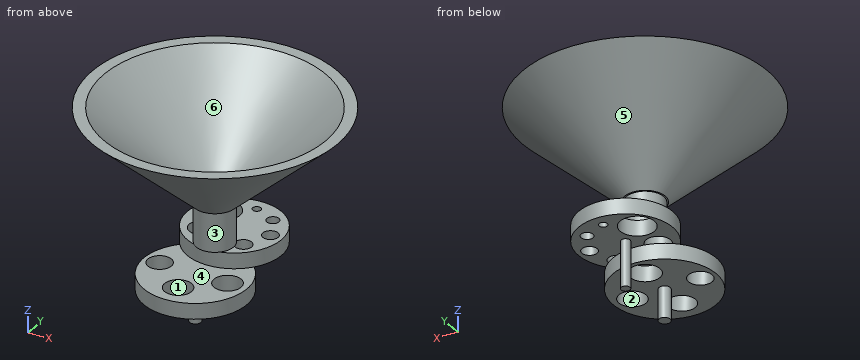
from build123d import *

# Parameters (mm, degrees)
SKETCH_1_R      = 60.353493774
SKETCH_1_R_2    = 5.249937669
SKETCH_1_R_3    = 7.709883183
SKETCH_1_R_4    = 9.776049215
SKETCH_1_R_5    = 10.682207241
SKETCH_1_R_6    = 12.535934249
SKETCH_1_R_7    = 15.691744865
SKETCH_1_R_8    = 21.933378779
EXTRUDE_1_DEPTH = 20
SKETCH_2_R      = 23.897110151
SKETCH_2_R_2    = 18.408818548
EXTRUDE_2_DEPTH = 50
SKETCH_5_R      = 5.758247264
EXTRUDE_3_DEPTH = 60
SKETCH_6_R      = 66.152888952
SKETCH_6_R_2    = 19.174469575
SKETCH_6_R_3    = 15.159489644
SKETCH_6_R_4    = 17.427329396
SKETCH_6_R_5    = 17.348205871
EXTRUDE_4_DEPTH = 20
SKETCH_7_R      = 7.266662744
EXTRUDE_5_DEPTH = 40


# Read off the part's stored shape, not the designer's step: 放样-薄件1
with BuildPart() as part:
    # 草图1 → 凸台-拉伸1 (new body)
    with BuildSketch(Plane.XY):
        Circle(SKETCH_1_R)
        with Locations((2.061161415, 43.884893492)):
            Circle(SKETCH_1_R_2, mode=Mode.SUBTRACT)
        with Locations((29.98052968, 32.080059931)):
            Circle(SKETCH_1_R_3, mode=Mode.SUBTRACT)
        with Locations((44.783416209, 2.661665183)):
            Circle(SKETCH_1_R_4, mode=Mode.SUBTRACT)
        with Locations((29.98052968, -30.316917465)):
            Circle(SKETCH_1_R_5, mode=Mode.SUBTRACT)
        with Locations((0, -40.999124706)):
            Circle(SKETCH_1_R_6, mode=Mode.SUBTRACT)
        with Locations((-28.294124885, -22.634406734)):
            Circle(SKETCH_1_R_7, mode=Mode.SUBTRACT)
        with Locations((-28.294124885, 21.774252854)):
            Circle(SKETCH_1_R_8, mode=Mode.SUBTRACT)
    extrude(amount=EXTRUDE_1_DEPTH)

    # 草图2 → 凸台-拉伸2 (add)
    with BuildSketch(Plane.XY.offset(20)):
        with Locations(Location((0, -40.999124706, 0), (0, 0, 171.88446927))):
            Circle(SKETCH_2_R)
        with Locations(Location((0, -40.999124706, 0), (0, 0, 154.797833564))):
            Circle(SKETCH_2_R_2, mode=Mode.SUBTRACT)
    extrude(amount=EXTRUDE_2_DEPTH)

    # 放样-薄件1 outline → 放样-薄件1 (revolve)
    with BuildSketch(Plane.XZ.offset(40.999124706)):
        Polygon((142.029499723, 190), (11.005834825, 70), (25.81180227, 70), (156.835467167, 190), align=None)
    revolve(axis=Axis((0, -40.999124706, 0), (0, 0, 1)))

    # 草图5 → 凸台-拉伸3 (add)
    with BuildSketch(Plane(origin=(0, 0, 0), x_dir=(-1, 0, 0), z_dir=(0, 0, -1))):
        with Locations(Location((0, 0, 0), (0, 0, 180))):
            Circle(SKETCH_5_R)
    extrude(amount=EXTRUDE_3_DEPTH)

    # 草图6 → 凸台-拉伸4 (add)
    with BuildSketch(Plane(origin=(0, 0, 0), x_dir=(-1, 0, 0), z_dir=(0, 0, -1))):
        with Locations(Location((0, -82.400396549, 0), (0, 0, 136.362104422))):
            Circle(SKETCH_6_R)
        with Locations(Location((0, -40.999124706, 0), (0, 0, 46.213976219))):
            Circle(SKETCH_6_R_2, mode=Mode.SUBTRACT)
        with Locations((45.85301636, -82.400396549)):
            Circle(SKETCH_6_R_3, mode=Mode.SUBTRACT)
        with Locations((-41.408908427, -82.400396549)):
            Circle(SKETCH_6_R_4, mode=Mode.SUBTRACT)
        with Locations((0, -118.765519068)):
            Circle(SKETCH_6_R_5, mode=Mode.SUBTRACT)
    extrude(amount=EXTRUDE_4_DEPTH)

    # 草图7 → 凸台-拉伸5 (add)
    with BuildSketch(Plane(origin=(0, 0, -20), x_dir=(-1, 0, 0), z_dir=(0, 0, -1))):
        with Locations((0, -82.400396549)):
            Circle(SKETCH_7_R)
    extrude(amount=EXTRUDE_5_DEPTH)


solid = part.part
The model under review builds one solid part; all positions refer to its coordinate system, in mm. Face numbers are marked on the shaded views. A direction names the side the tool comes from. Coordinates: 2 decimals unless noted, no trailing zeros. Loops run counter-clockwise (first coordinate to the right, second up) from the corner with the lowest first, then second, coordinate; pieces in that order, holes last.
(1) Consider section A-A, the plane y = -110. Give the number of separate pieces and of enclosed holes in the cut face, plus the area to 3 significant figures.
Determined:
separate pieces: 3
enclosed holes: 0
area: 5,400 mm2
(2) Tool access review of the marked faces 5 and 6: name each direction out of +Z, -Z, +X, -X, +Y, -Y from which nothing blocks a thin tool from reaching the whole face with its end or side.
Determined:
face 5: none
face 6: +Z
(3) Consider section C-C, the plane z = 159. Give the boundary of the cut face in (x, y), plus the area to 3 significant figures.
Determined:
outline: circle Ø245.98 at (0, -41); hole circle Ø216.36 at (0, -41)
area: 10,800 mm2
(4) Insertion check: P1, Ø3, axis at y = 5.5, z = 101.5, coming from the -X side; P2, Ø5, axis at y = 8, z = 103.5, coming from the -X side; P3, Ø3, axis at y = -62.5, z = 119.5, coming from the -X side. Each pin has a flat end and moves straight along its axis. Give the tip position at first contact, or say it passes through.
Determined:
P1: stops at x = -41.29
P2: stops at x = -43.75
P3: stops at x = -78.66
(5) Draft analysis for pull direction Y (two halves, no side actions). For the marked faces 1, 2, 3 and 4, state which applies: +Y half, -Y half, draft (parallel to the pull), parting line (faces both ways), or undercut.
Determined:
face 1: undercut
face 2: undercut
face 3: parting line
face 4: draft
(6) Consider section B-B, the plane z = -34.5. Give the boundary of the cut face in (x, y), plus the area to 3 significant figures.
Determined:
outline: circle Ø14.53 at (0, -82.4); circle Ø11.52 at (0, 0)
area: 270 mm2
(7) Wall thickness on L1, parallel to Y at x = -94.5, z = 160.5; L2, parallel to Z at x = -0.5, y = -56; L3, parallel to Z at x = 32, y = -39.5: over which ranges is each line inside the solid? List them lowest first.
Determined:
L1: y = -122.25 to -96.95, 14.95 to 40.25
L2: z = 0 to 20, 70 to 73.67
L3: z = -20 to 0, 75.7 to 89.26
